CAD build for the part. Positions are in the model's coordinates, mm. Coordinates: 2 decimals unless noted, no trailing zeros. Order: outer loops, then holes, each group sorted by start corner. A loop starts at its lowest first (then second) coordinate and runs counter-clockwise, first axis right, second up. Notation, with made-up numbers: M 23.5,59.5 L 51.5,59.5 A31 ccw 51.5,86.5 Z; hole C 85.25,20 d3. An arc over 180 degrees is marked long. One line per item, written item: value.
from build123d import *

# Parameters (mm, degrees)
SKETCH1_R           = 1.75
BOSS_EXTRUDE1_DEPTH = 4


with BuildPart() as part:
    # Sketch1 → Boss-Extrude1 (new body)
    with BuildSketch(Plane(origin=(0, 0, 0), x_dir=(1, 0, 0), z_dir=(0, 1, 0))):
        with BuildLine():
            Line((-28.2, -67), (28.2, -67))
            Line((28.2, -67), (28.2, -29.8))
            Line((28.2, -29.8), (31.2, -29.8))
            Line((31.2, -29.8), (31.2, -9))
            ThreePointArc((31.2, -9), (33.543145751, -3.343145751), (39.2, -1))
            Line((39.2, -1), (50, -1))
            Line((50, -1), (50, 67.103600519))
            ThreePointArc((50, 67.103600519), (49.522172621, 69.827002629), (48.145770237, 72.225075716))
            Line((48.145770237, 72.225075716), (25, 100))
            Line((25, 100), (15, 100))
            ThreePointArc((15, 100), (13.585786438, 99.414213562), (13, 98))
            Line((13, 98), (13, 82))
            Line((13, 82), (-13, 82))
            Line((-13, 82), (-13, 98))
            ThreePointArc((-13, 98), (-13.585786438, 99.414213562), (-15, 100))
            Line((-15, 100), (-25, 100))
            Line((-25, 100), (-48.145770237, 72.225075716))
            ThreePointArc((-48.145770237, 72.225075716), (-49.522172621, 69.827002629), (-50, 67.103600519))
            Line((-50, 67.103600519), (-50, -1))
            Line((-50, -1), (-39.2, -1))
            ThreePointArc((-39.2, -1), (-33.543145751, -3.343145751), (-31.2, -9))
            Line((-31.2, -9), (-31.2, -29.8))
            Line((-31.2, -29.8), (-28.2, -29.8))
            Line((-28.2, -29.8), (-28.2, -67))
        make_face()
        with Locations((18, 0)):
            Circle(SKETCH1_R, mode=Mode.SUBTRACT)
        with Locations((-18, 0)):
            Circle(SKETCH1_R, mode=Mode.SUBTRACT)
        with Locations((29, 64)):
            Circle(SKETCH1_R, mode=Mode.SUBTRACT)
        with Locations((-29, 64)):
            Circle(SKETCH1_R, mode=Mode.SUBTRACT)
        with BuildLine():
            Line((-13, 3), (13, 3))
            ThreePointArc((13, 3), (15.121320344, 3.878679656), (16, 6))
            Line((16, 6), (16, 62))
            ThreePointArc((16, 62), (15.121320344, 64.121320344), (13, 65))
            Line((13, 65), (-13, 65))
            ThreePointArc((-13, 65), (-15.121320344, 64.121320344), (-16, 62))
            Line((-16, 62), (-16, 6))
            ThreePointArc((-16, 6), (-15.121320344, 3.878679656), (-13, 3))
        make_face(mode=Mode.SUBTRACT)
        with BuildLine():
            Line((-4, -51), (4, -51))
            ThreePointArc((4, -51), (8, -55), (4, -59))
            Line((4, -59), (-4, -59))
            ThreePointArc((-4, -59), (-8, -55), (-4, -51))
        make_face(mode=Mode.SUBTRACT)
        Polygon((28.160862107, 92.770455614), (41.6047345, 76.637808743), (31.464213609, 68.187374667), (18.020341216, 84.320021539), align=None, mode=Mode.SUBTRACT)
    extrude(amount=BOSS_EXTRUDE1_DEPTH)


solid = part.part
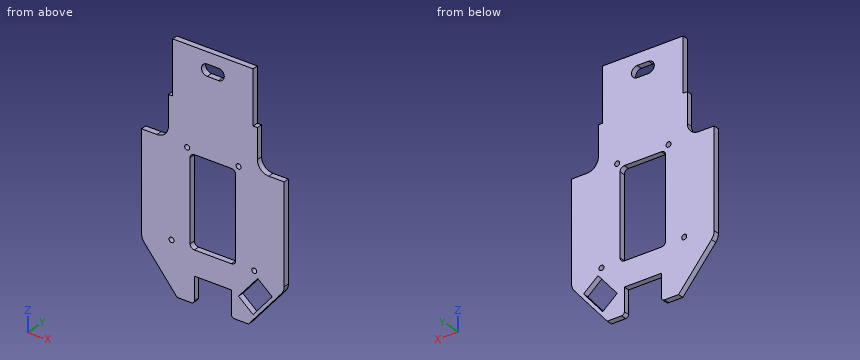
Q1. Slice it at C-C (y = 1.7). Give the number of separate pieces and of enclosed holes in the cut face, plus the area to 3 significant figures.
Recorded:
separate pieces: 1
enclosed holes: 7
area: 10,400 mm^2
Q2. Drill centre lines: line 1 along X through (y, z) = (2.25, 0); line 2 along X through (y, z) = (3.35, -58); line 3 along X through (y, z) = (2.95, -64). Where is each one in solid material? Low to high.
Recorded:
line 1: x = -50 to -19.75, -16.25 to 16.25, 19.75 to 50
line 2: x = -50 to -16, 16 to 50
line 3: x = -50 to -30.75, -27.25 to -15.24, 15.24 to 27.25, 30.75 to 50
Q3. Slice it at A-A (z = 55). List the corners of the cut face in (x, y).
Recorded:
outline: M -28.2,0 L -8,0 L -8,4 L -28.2,4 Z; M 8,0 L 28.2,0 L 28.2,4 L 8,4 Z
Q4. Slice it at B-B (x = 37). List the corners of the cut face in (y, z), plus the area to 3 significant figures.
Recorded:
outline: M 0,-85.6 L 4,-85.6 L 4,-82.16 L 0,-82.16 Z; M 0,-72.8 L 4,-72.8 L 4,1.31 L 0,1.31 Z
area: 310 mm^2
Q5. Slice it at D-D (x = -34). List the corners of the cut face in (y, z), plus the area to 3 significant figures.
Recorded:
outline: M 0,-89.2 L 4,-89.2 L 4,2.92 L 0,2.92 Z
area: 368 mm^2
Q6. Pin check, flat tips, straight feed: pin 1 Ø1 at (x, z) = (27, 29) entering from -Y; pin 2 Ø1.2 at (x, y) = (-44.5, 3) entering from +Z; pin 3 Ø1.2 at (x, y) = (-0.5, 1) entering from -Z; pin 4 Ø2 at (y, z) = (3, -75) entering from +X. Stop position of each tip, or through.
Recorded:
pin 1: stops at y = 0
pin 2: stops at z = 1
pin 3: stops at z = -82
pin 4: stops at x = 46.67
